from build123d import *

# Parameters (mm, degrees)
SKETCH1_R           = 8.5
BOSS_EXTRUDE1_DEPTH = 5.45
SKETCH2_R           = 1
CUT_EXTRUDE1_DEPTH  = 5.45
SKETCH3_R           = 2.5
BOSS_EXTRUDE2_DEPTH = 18.6
SKETCH6_R           = 2.1
CUT_EXTRUDE2_DEPTH  = 1.2
SKETCH7_R           = 4.5
CUT_EXTRUDE3_DEPTH  = 2


with BuildPart() as part:
    # Sketch1 → Boss-Extrude1 (new body)
    with BuildSketch(Plane.XY):
        Circle(SKETCH1_R)
    extrude(amount=BOSS_EXTRUDE1_DEPTH)

    # Sketch2 → Cut-Extrude1 (cut)
    with BuildSketch(Plane.XY.offset(5.45)):
        with Locations((0, 6)):
            Circle(SKETCH2_R)
        with Locations((5.196152423, -3)):
            Circle(SKETCH2_R)
        with Locations((-5.196152423, -3)):
            Circle(SKETCH2_R)
    extrude(amount=-CUT_EXTRUDE1_DEPTH, mode=Mode.SUBTRACT)

    # Sketch3 → Boss-Extrude2 (add)
    with BuildSketch(Plane.XY.offset(5.45)):
        Circle(SKETCH3_R)
    extrude(amount=BOSS_EXTRUDE2_DEPTH)

    # Sketch6 → Cut-Extrude2 (cut)
    with BuildSketch(Plane.XY.offset(5.45)):
        with Locations((5.196152423, -3)):
            Circle(SKETCH6_R)
        with Locations((0, 6)):
            Circle(SKETCH6_R)
        with Locations((-5.196152423, -3)):
            Circle(SKETCH6_R)
    extrude(amount=-CUT_EXTRUDE2_DEPTH, mode=Mode.SUBTRACT)

    # Sketch7 → Cut-Extrude3 (cut)
    with BuildSketch(Plane(origin=(0, 0, 0), x_dir=(-1, 0, 0), z_dir=(0, 0, -1))):
        Circle(SKETCH7_R)
    extrude(amount=-CUT_EXTRUDE3_DEPTH, mode=Mode.SUBTRACT)


solid = part.part
Verification items for the finished model (mm, model axes). A direction names the side the tool comes from. Coordinates: 2 decimals unless noted, no trailing zeros. Write each loop counter-clockwise with the first axis right and the second up, starting at its lowest first coordinate (ties: lowest second). Pieces come first, ordered by that corner, then holes. Notation, with made-up numbers: (-16, -23) -> (30, -23) arc R17 ccw to (30, -12) -> close; hole circle Ø5 at (83.25, 79.5). An arc over 180 degrees is marked (long way). One line per item, written item: value. Start each with the question number.
Q1. Cross-section at D-D on y = 0. Enter the section's corners in (x, z).
Q2. Thickness scan on L1, parallel to Y at x = 0, z = 1.35; L2, parallel to Y at x = 0, z = 4.75; L3, parallel to Z at x = -3.75, y = 2. Record the ranges inside material, lowest first. Write a range as from..to.
Q3. Mould release check, pull along Y, two halves, no side actions. Record for faces 1 (the cylindrical face through (-5.99, -3.61, 2.15)), 2 (the flat face through (2, -2, 5.45)), 3 (the cylindrical face through (-0.54, -2.44, 14.62)): pulls with the +Y half, pulls with the -Y half, needs draft (parallel to the pull), parting line crosses it, or undercut.
Q4. Cross-section at A-A on x = 0. Enter the section's corners in (y, z).
Q5. Go/stop test with flat-tipped pins: P1, Ø8, axis at y = -4.5, z = 7.5, coming from the +X side; P2, Ø4.5, axis at x = 0, y = 6, coming from the +Z side; P3, Ø3, axis at x = 2.5, y = -1, coming from the -Z side; P4, Ø3.5, axis at x = 0, y = 6, coming from the -Z side. Record where each tip stops, or that it passes through.
Q6. Cross-section at C-C on y = 6. Enter the section's corners in (x, z), and give its area (3 significant figures).
Q7. Access from +Z, -Z, +X, -X, +Y, -Y to the whole of each face (thin tool, end or side, straight path). Record for faces 4 (the flat face through (6, -4, 4.25)), 5 (the cylindrical face through (4.197, -2.956, 2.155)), 6 (the flat face through (0, 0, 2)).
Q8. Cross-section at B-B on z = 1.5. Enter the section's corners in (x, y), and give its area (3 significant figures).
Checked values:
1. outline: (-8.5, 0) -> (-4.5, 0) -> (-4.5, 2) -> (4.5, 2) -> (4.5, 0) -> (8.5, 0) -> (8.5, 5.45) -> (2.5, 5.45) -> (2.5, 24.05) -> (-2.5, 24.05) -> (-2.5, 5.45) -> (-8.5, 5.45) -> close
2. L1: y = -8.5..-4.5, 4.5..5, 7..8.5
2. L2: y = -8.5..3.9, 8.1..8.5
2. L3: z = 2..5.45
3. face 1: undercut
3. face 2: needs draft
3. face 3: parting line crosses it
4. outline: (-8.5, 0) -> (-4.5, 0) -> (-4.5, 2) -> (4.5, 2) -> (4.5, 0) -> (5, 0) -> (5, 4.25) -> (3.9, 4.25) -> (3.9, 5.45) -> (2.5, 5.45) -> (2.5, 24.05) -> (-2.5, 24.05) -> (-2.5, 5.45) -> (-8.5, 5.45) -> close; (7, 0) -> (8.5, 0) -> (8.5, 5.45) -> (8.1, 5.45) -> (8.1, 4.25) -> (7, 4.25) -> close
5. P1: stops at x = 8.43
5. P2: stops at z = 5.45
5. P3: stops at z = 2
5. P4: stops at z = 0
6. outline: (-6.02, 0) -> (-1, 0) -> (-1, 4.25) -> (-2.1, 4.25) -> (-2.1, 5.45) -> (-6.02, 5.45) -> close; (1, 0) -> (6.02, 0) -> (6.02, 5.45) -> (2.1, 5.45) -> (2.1, 4.25) -> (1, 4.25) -> close
6. area: 52.1 mm²
7. face 4: +Z
7. face 5: +Z, -Z
7. face 6: -Z
8. outline: circle Ø17 at (0, 0); hole circle Ø2 at (-5.2, -3); hole circle Ø9 at (0, 0); hole circle Ø2 at (0, 6); hole circle Ø2 at (5.2, -3)
8. area: 154 mm²
